Verification items for this drawing (mm, ordinates from the low corner). A direction names the side the tool comes from. Round coordinates to 2 decimals unless told otherwise and drop trailing zeros. Order: outer loops, then holes, each group sorted by start corner. A loop starts at its lowest first (then second) coordinate and runs counter-clockwise, first axis right, second up. Notation, with made-up numbers: (17.5, 56.5) -> (34.5, 56.5) arc R16 cw to (34.5, 71.5) -> close; hole circle Ø9 at (-28.75, 37). An arc over 180 degrees is marked (long way). Use a Markdown table: item, result. Add a question column.
Item 1: Sectioned sample at B-B, the plane x = 128. Record the cut outline in (y, z), and give its area (3 significant figures).
Item 2: Sectioned sample at A-A, the plane y = 23.5. Record the cut outline in (x, z).
Item 3: Set-up check for the marked faces 1, 2 and 3: record each of +Z, -Z, +X, -X, +Y, -Y from which the full face is reachable in a straight line by a thin tool's end or side.
Item 4: Sectioned sample at C-C, the plane z = 17.5. Record the cut outline in (x, y), and give its area (3 significant figures).
Item 5: Gauge pin test, flat ends, axial feed: pin 1 Ø1 at (y, z) = (130, 13.5) entering from +X; pin 2 Ø1.6 at (y, z) = (135.5, 12.5) entering from -X; pin 3 Ø6 at (x, y) = (177.5, 51) entering from -Z. Record the tip position at first contact, or that the pin passes through.
Item 6: Sectioned sample at D-D, the plane y = 70. Record the cut outline in (x, z).
Item 7: Material ranges on probe 1 along X at (y, z) = (142, 11.25); probe 2 along Z at (x, y) = (259.5, 134); probe 3 along Z at (x, y) = (195, 81.5), recorded low to high. Write a range as [from, to].
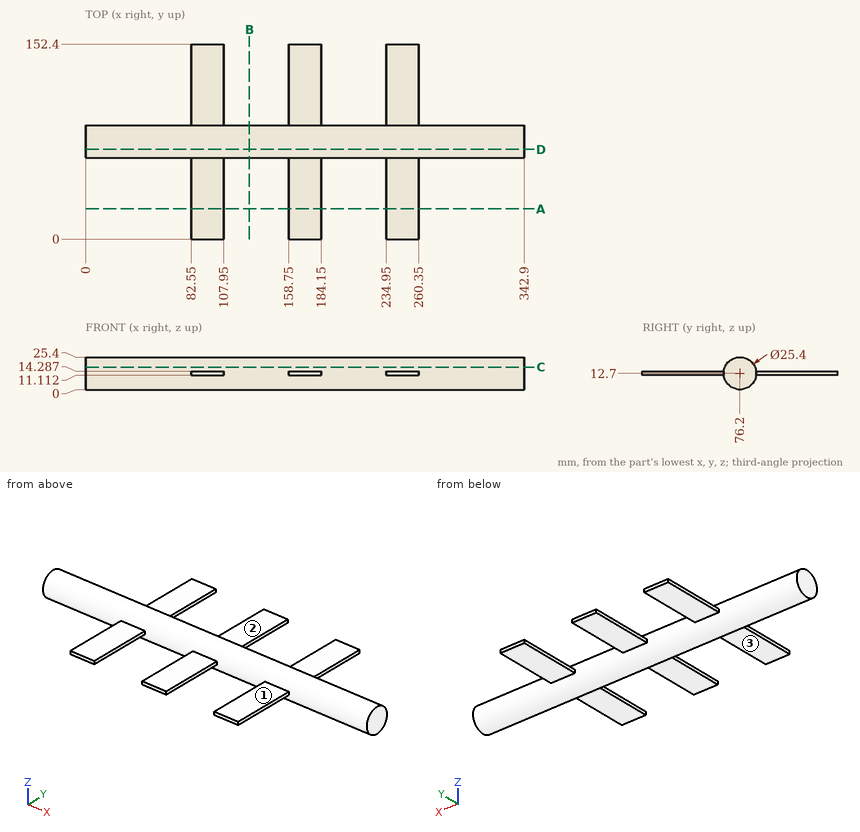
Found:
| question | item | result |
|---|---|---|
| 1 | outline | circle Ø25.4 at (76.2, 12.7) |
| 1 | area | 507 mm2 |
| 2 | outline | (82.55, 11.11) -> (107.95, 11.11) -> (107.95, 14.29) -> (82.55, 14.29) -> close; (158.75, 11.11) -> (184.15, 11.11) -> (184.15, 14.29) -> (158.75, 14.29) -> close; (234.95, 11.11) -> (260.35, 11.11) -> (260.35, 14.29) -> (234.95, 14.29) -> close |
| 3 | face 1 | +Z, +X, -X, -Y |
| 3 | face 2 | +Z, +X, -X, +Y |
| 3 | face 3 | -Z, +X, -X, -Y |
| 4 | outline | (0, 64.44) -> (342.9, 64.44) -> (342.9, 87.96) -> (0, 87.96) -> close |
| 4 | area | 8,060 mm2 |
| 5 | pin 1 | stops at x = 260.35 |
| 5 | pin 2 | stops at x = 82.55 |
| 5 | pin 3 | stops at z = 11.11 |
| 6 | outline | (0, 1.62) -> (342.9, 1.62) -> (342.9, 23.78) -> (0, 23.78) -> close |
| 7 | probe 1 | x = [82.55, 107.95], [158.75, 184.15], [234.95, 260.35] |
| 7 | probe 2 | z = [11.11, 14.29] |
| 7 | probe 3 | z = [1.16, 24.24] |
